The listing builds one solid part. Answer for the finished solid, in the listing's coordinates (mm). A direction names the side the tool comes from. Coordinates: 2 decimals unless noted, no trailing zeros. Write each loop counter-clockwise with the first axis right and the second up, starting at its lowest first coordinate (ties: lowest second). Pieces come first, ordered by that corner, then holes. Notation, with made-up numbers: M -12.5,44 L 43.5,44 A18 ccw 43.5,50 Z; hole C -11.75,-0.75 d9. An arc over 180 degrees is marked long. Put each result on its own line as item: value. Start each with the question number.
```python
from build123d import *

# Parameters (mm, degrees)
BOSS_EXTRUDE1_DEPTH = 19.05
SKETCH2_W           = 8.554162714
SKETCH2_H           = 38.1
BOSS_EXTRUDE2_DEPTH = 4.763405733
SKETCH3_R           = 4.277081357
BOSS_EXTRUDE3_DEPTH = 19.05
CUT_EXTRUDE1_REACH  = 86.087
CUT_EXTRUDE2_REACH  = 86.087


with BuildPart() as part:
    # Sketch1 → Boss-Extrude1 (new body)
    with BuildSketch(Plane.YZ):
        Polygon((0, 0), (0, 50.133536148), (26.05701333, 50.133536148), (26.05701333, 44.11057508), (0.67733333, 44.11057508), (0.67733333, 6.03597508), (64.08589333, 6.03597508), (64.08589333, 44.11057508), (38.70621333, 44.11057508), (38.70621333, 50.133536148), (64.76322666, 50.133536148), (64.76322666, 0), align=None)
    extrude(amount=BOSS_EXTRUDE1_DEPTH)

    # Sketch2 → Boss-Extrude2 (add)
    with BuildSketch(Plane(origin=(0, 0, 0), x_dir=(0, -1, 0), z_dir=(-1, 0, 0))):
        with Locations((-32.38161333, -13.01402492)):
            Rectangle(SKETCH2_W, SKETCH2_H)
    extrude(amount=BOSS_EXTRUDE2_DEPTH)

    # Sketch3 → Boss-Extrude3 (add)
    with BuildSketch(Plane.YZ):
        with Locations(Location((32.38161333, -27.786943563, 0), (0, 0, 270))):
            Circle(SKETCH3_R)
    extrude(amount=BOSS_EXTRUDE3_DEPTH)

    # Sketch5 → Cut-Extrude1 (cut, up to next)
    with BuildSketch(Plane.YZ, mode=Mode.PRIVATE) as cut_extrude1_sk1:
        with BuildLine():
            Line((32.38161333, -32.06402492), (36.658694687, -32.06402492))
            Line((36.658694687, -32.06402492), (36.658694687, -27.786943563))
            ThreePointArc((36.658694687, -27.786943563), (35.405966561, -30.811296794), (32.38161333, -32.06402492))
        make_face()
    cut_extrude1_tool1 = extrude(cut_extrude1_sk1.sketch, amount=-CUT_EXTRUDE1_REACH, mode=Mode.PRIVATE) & part.part
    add(cut_extrude1_tool1.solids().sort_by_distance((0, 35.703332, -31.108662))[0], mode=Mode.SUBTRACT)

    # Sketch6 → Cut-Extrude2 (cut, up to next)
    with BuildSketch(Plane.YZ, mode=Mode.PRIVATE) as cut_extrude2_sk1:
        with BuildLine():
            Line((28.104531973, -27.786943563), (28.104531973, -32.06402492))
            Line((28.104531973, -32.06402492), (32.38161333, -32.06402492))
            ThreePointArc((32.38161333, -32.06402492), (29.357260099, -30.811296794), (28.104531973, -27.786943563))
        make_face()
    cut_extrude2_tool1 = extrude(cut_extrude2_sk1.sketch, amount=-CUT_EXTRUDE2_REACH, mode=Mode.PRIVATE) & part.part
    add(cut_extrude2_tool1.solids().sort_by_distance((0, 29.059895, -31.108662))[0], mode=Mode.SUBTRACT)


solid = part.part
```
1) A cutting plane is placed at D-D on x = -1.25. Write down the section's boundary in (y, z), then the cut area to 3 significant figures.
2) A cutting plane is placed at C-C on y = 50.5. Write down the section's boundary in (x, z).
3) Given pin 1 Ø5 at (x, z) = (-1.5, -13) entering from -Y; pin 2 Ø9.5 at (x, y) = (11.5, 17) entering from -Z; pin 3 Ø4 at (y, z) = (29.5, -12.5) entering from +X; pin 4 Ø6 at (y, z) = (10, 39) entering from -X, each flat-ended and moving along its own axis, determine where each tip first touches the part or whether it passes through.
4) Determine the mould class of faces 1 (the face through (9, 26.057, 47)), 2 (the face through (9, 52, 50.134)), 3 (the face through (10, 33, 6.036)) for opening direction Z: +Z half, -Z half, draft (parallel to the pull), parting line (faces both ways), or undercut.
5) A cutting plane is placed at B-B on z = 34.5. Write down the section's boundary in (x, y).
6) Straight lines are drawn through the part: probe 1 along Z at (x, y) = (4.25, 22); probe 2 along Y at (x, z) = (5.5, 16.5); probe 3 along X at (y, z) = (47.5, 5). For each, find the intervals that lie inside material, in ascending order.
7) For faces 4 (the face through (-2, 28.105, -11)), 5 (the face through (9, 52, 44.111)), 6 (the face through (0, 64.3, 25.2)), 7 (the face through (9, 38.706, 47)), 8 (the face through (19.05, 30, 5)), determine the directions among +Z, -Z, +X, -X, +Y, -Y from which every point of the face is accessible in a straight line to the end or side of a thin tool.
8) A cutting plane is placed at A-A on x = 13.75. Write down the section's boundary in (y, z), then the cut area to 3 significant figures.
Answers follow:
1. outline: M 28.1,-27.79 A4.28 ccw 36.66,-27.79 L 36.66,6.04 L 28.1,6.04 Z
1. area: 318 mm²
2. outline: M 0,0 L 19.05,0 L 19.05,6.04 L 0,6.04 Z; M 0,44.11 L 19.05,44.11 L 19.05,50.13 L 0,50.13 Z
3. pin 1: stops at y = 28.1
3. pin 2: stops at z = 0
3. pin 3: stops at x = 0
3. pin 4: passes through
4. face 1: draft
4. face 2: +Z half
4. face 3: undercut
5. outline: M 0,0 L 19.05,0 L 19.05,0.68 L 0,0.68 Z; M 0,64.09 L 19.05,64.09 L 19.05,64.76 L 0,64.76 Z
6. probe 1: z = 0 to 6.04, 44.11 to 50.13
6. probe 2: y = 0 to 0.68, 64.09 to 64.76
6. probe 3: x = 0 to 19.05
7. face 4: +Z, -Z, -X, -Y
7. face 5: +X, -X
7. face 6: +Z, -Z, -X, +Y
7. face 7: +Z, +X, -X
7. face 8: +Z, -Z, +X, +Y, -Y
8. outline: M 0,0 L 64.76,0 L 64.76,50.13 L 38.71,50.13 L 38.71,44.11 L 64.09,44.11 L 64.09,6.04 L 0.68,6.04 L 0.68,44.11 L 26.06,44.11 L 26.06,50.13 L 0,50.13 Z; C 32.38,-27.79 d8.55
8. area: 814 mm²
